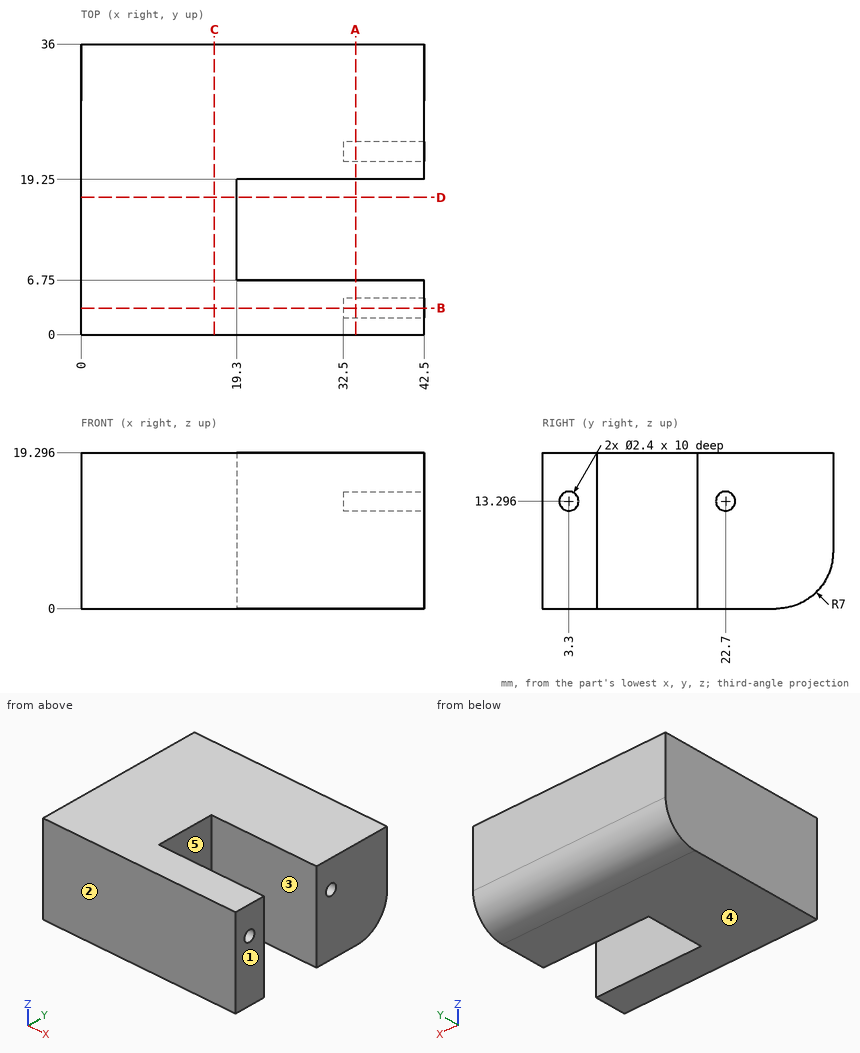
Geometry check sheet. Reference: drawing and pictorial views, mm from the part's lowest x, y, z. A direction names the side the tool comes from. Round coordinates to 2 decimals unless told otherwise and drop trailing zeros. Loops run counter-clockwise (first coordinate to the right, second up) from the corner with the lowest first, then second, coordinate; pieces in that order, holes last. Notation, with made-up numbers: (-19.5, 70) - (6.5, 70) arc R13 ccw to (6.5, 85) - close; hole circle Ø11 at (12.5, -29.5). An arc over 180 degrees is marked (long way). Write item = value, one per line. Start each with the question number.
Q1. Access from +Z, -Z, +X, -X, +Y, -Y to the whole of each face (thin tool, end or side, straight path). Record for the marked faces 4 and 5.
Q2. Depth check by flat-ended pin: P1, Ø1, axis at x = 27, y = 8.5, coming from the +Z side; P2, Ø1.2, axis at y = 3, z = 13, coming from the +X side. Enter the tip coordinate at first touch or a pass-through.
Q3. Section check B-B (y = 3.3). Record the boundary of the cut face in (x, z), plus the area to 3 significant figures.
Q4. Thickness scan on L1, parallel to Y at x = 20, z = 18.75; L2, parallel to Z at x = 36.5, y = 22.7; L3, parallel to X at y = 10, z = 2. Record the ranges inside material, lowest first.
Q5. Section check D-D (y = 17). Record the boundary of the cut face in (x, z), plus the area to 3 significant figures.
Q6. Section check A-A (x = 34). Record the boundary of the cut face in (y, z).
Q7. Release check for a two-part mould opening along Y. For the marked faces 1, 2 and 3 record: pulls with the +Y half, pulls with the -Y half, needs draft (parallel to the pull), parting line crosses it, or undercut.
Q8. Section check C-C (x = 16.5). Record the boundary of the cut face in (y, z), plus the area to 3 significant figures.
Derived:
q1.face_4 = -Z, +X, -X, +Y, -Y
q1.face_5 = +Z, -Z, +X
q2.P1 = through
q2.P2 = 32.5
q3.outline = (0, 0) - (42.5, 0) - (42.5, 12.1) - (32.5, 12.1) - (32.5, 14.5) - (42.5, 14.5) - (42.5, 19.3) - (0, 19.3) - close
q3.area = 796 mm^2
q4.L1 = 0 to 6.75, 19.25 to 36
q4.L2 = 0 to 12.1, 14.5 to 19.3
q4.L3 = 0 to 19.3
q5.outline = (0, 0) - (19.3, 0) - (19.3, 19.3) - (0, 19.3) - close
q5.area = 372 mm^2
q6.outline = (0, 0) - (6.75, 0) - (6.75, 19.3) - (0, 19.3) - close; (19.25, 0) - (29, 0) arc R7 ccw to (36, 7) - (36, 19.3) - (19.25, 19.3) - close; hole circle Ø2.4 at (3.3, 13.3); hole circle Ø2.4 at (22.7, 13.3)
q7.face_1 = needs draft
q7.face_2 = pulls with the -Y half
q7.face_3 = undercut
q8.outline = (0, 0) - (29, 0) arc R7 ccw to (36, 7) - (36, 19.3) - (0, 19.3) - close
q8.area = 684 mm^2
